from build123d import *

# Parameters (mm, degrees)
PAD_DEPTH   = 3
FILLET_R    = 3
FILLET001_R = 1
FILLET002_R = 5
FILLET003_R = 3


with BuildPart() as part:
    # Sketch → Pad (new body)
    with BuildSketch(Plane.XY):
        Polygon((0, 0), (30.749545, 0), (30.749545, 2), (29.374773, 5), (25.374773, 5), (24, 2), (2, 2), (2, 17.5), (24, 17.5), (25.374773, 14.5), (29.374773, 14.5), (30.749545, 17.5), (30.749545, 19.5), (0, 19.5), align=None)
    extrude(amount=PAD_DEPTH)

    # Fillet
    fillet_edges = [part.edges().sort_by_distance(p)[0] for p in [
        (29.374773, 5, 1.5),
        (29.374773, 14.5, 1.5),
    ]]
    fillet(fillet_edges, radius=FILLET_R)

    # Fillet001
    fillet001_edges = [part.edges().sort_by_distance(p)[0] for p in [
        (30.749545, 2, 1.5),
        (30.749545, 0, 1.5),
        (30.749545, 19.5, 1.5),
        (30.749545, 17.5, 1.5),
    ]]
    fillet(fillet001_edges, radius=FILLET001_R)

    # Fillet002
    fillet002_edges = [part.edges().sort_by_distance(p)[0] for p in [
        (2, 2, 1.5),
        (2, 17.5, 1.5),
    ]]
    fillet(fillet002_edges, radius=FILLET002_R)

    # Fillet003
    fillet003_edges = [part.edges().sort_by_distance(p)[0] for p in [
        (0, 0, 1.5),
        (0, 19.5, 1.5),
    ]]
    fillet(fillet003_edges, radius=FILLET003_R)


solid = part.part
Build history of the part. All positions in model axes, mm. A direction names the side the tool comes from. Coordinates: 2 decimals unless noted, no trailing zeros. Order: outer loops, then holes, each group sorted by start corner. A loop starts at its lowest first (then second) coordinate and runs counter-clockwise, first axis right, second up. Notation, with made-up numbers: (37, 24.25) - (80, 24.25) arc R27 ccw to (80, 52.25) - close; hole circle Ø10 at (70, 3). An arc over 180 degrees is marked (long way). Write item = value, one per line. Start each with the question number.
1) Wall check: line 1 along Y through (x, z) = (16.5, 1.3); line 2 along Y through (x, z) = (4, 0.7); line 3 along X through (y, z) = (9, 1.95). Give the ranges that are in metal, low to high. Write a range as from..to.
2) Saw through at D-D on x = 5. Write the cut outline in (y, z).
3) Saw through at A-A on x = 21. Write the cut outline in (y, z).
4) Two-plate mould, pull along Y, no slides. Class faces 1 (the face through (0.86, 18.6, 1.52)), 2 (the face through (0.9, 0.86, 1.52)), 3 (the face through (26, 14.5, 1)), 4 (the face through (13, 18, 3)): pulls with the +Y half, pulls with the -Y half, needs draft (parallel to the pull), parting line crosses it, or undercut.
5) Flat gauge pin, fed straight in: pin 1 Ø4 at (x, y) = (26.5, 17) entering from -Z. Where does the tip first touch, or does it go through?
6) 3-axis set-ups, long thin cutter, end or side, ignore diameter. For faces 5 (the face through (24.697, 3.521, 1.479)), 6 (the face through (30.42, 2.72, 1.48)), 7 (the face through (0, 10, 1)): which of +Z, -Z, +X, -X, +Y, -Y reach the whole face in a straight line?
7) Saw through at B-B on z = 1.2. Write the cut outline in (x, y).
8) Saw through at C-C on y = 10.25. Write the cut outline in (x, z).
From the geometry:
q1.line_1 = 0..2, 17.5..19.5
q1.line_2 = 0..3, 16.5..19.5
q1.line_3 = 0..2
q2.outline = (0, 0) - (2.42, 0) - (2.42, 3) - (0, 3) - close; (17.08, 0) - (19.5, 0) - (19.5, 3) - (17.08, 3) - close
q3.outline = (0, 0) - (2, 0) - (2, 3) - (0, 3) - close; (17.5, 0) - (19.5, 0) - (19.5, 3) - (17.5, 3) - close
q4.face_1 = pulls with the +Y half
q4.face_2 = pulls with the -Y half
q4.face_3 = undercut
q4.face_4 = needs draft
q5.pin_1 = 0
q6.face_5 = +Z, -Z
q6.face_6 = +Z, -Z, +X
q6.face_7 = +Z, -Z, -X, +Y, -Y
q7.outline = (0, 3) arc R3 ccw to (3, 0) - (29.75, 0) arc R1 ccw to (30.75, 1) - (30.75, 1.78) arc R1 ccw to (30.66, 2.2) - (30.18, 3.25) arc R3 ccw to (27.45, 5) - (25.37, 5) - (24, 2) - (7, 2) arc R5 cw to (2, 7) - (2, 12.5) arc R5 cw to (7, 17.5) - (24, 17.5) - (25.37, 14.5) - (27.45, 14.5) arc R3 ccw to (30.18, 16.25) - (30.66, 17.3) arc R1 ccw to (30.75, 17.72) - (30.75, 18.5) arc R1 ccw to (29.75, 19.5) - (3, 19.5) arc R3 ccw to (0, 16.5) - close
q8.outline = (0, 0) - (2, 0) - (2, 3) - (0, 3) - close
